Work out the finished part from the listing and answer in its coordinate system (mm). Round coordinates to 2 decimals unless told otherwise and drop trailing zeros. Loops run counter-clockwise (first coordinate to the right, second up) from the corner with the lowest first, then second, coordinate; pieces in that order, holes last. Notation, with made-up numbers: (15.5, 12.25) - (54.5, 12.25) arc R22 ccw to (54.5, 29.25) - close; hole circle Ø4 at (-24, 72.5). An arc over 180 degrees is marked (long way). Answer as CSV lines item,"result". Start each with the question number.
Q1. Section A-A on x = 35.5 is taken. Write down the section's boundary in (y, z), then the cut area to 3 significant figures.
Q2. Section B-B on z = 0.9 is taken. Write down the section's boundary in (x, y), then the cut area to 3 significant figures.
Q3. Section C-C on y = 0 is taken. Write down the section's boundary in (x, z).
Q4. Straight lines are drawn through the part: L1, parallel to Y at x = 21.5, z = 0.85; L2, parallel to X at y = -3.5, z = 1.1; L3, parallel to X at y = 11.5, z = 0.85. For each, find the intervals that lie inside material, in ascending order. Write a range as [from, to].
```python
from build123d import *

# Parameters (mm, degrees)
F0_W     = 87
F0_H     = 59
F1_DEPTH = 2
F2_R     = 17.5
F3_DEPTH = 25
F4_DEPTH = 20
F5_R     = 4


with BuildPart() as f1:
    # F0 (on Top) → F1 (new body)
    with BuildSketch(Plane.XY):
        Rectangle(F0_W, F0_H)
    extrude(amount=F1_DEPTH)

    # F2 (on face) → F3 (cut)
    with BuildSketch(Plane.XY.offset(2)):
        with Locations((21.5, 0)):
            Circle(F2_R)
    extrude(amount=-F3_DEPTH, mode=Mode.SUBTRACT)

    # F4 (add): a face of the model
    f4_faces = [f1.faces().sort_by_distance(p)[0] for p in [
        (-43.5, 0, 1),
    ]]
    extrude(f4_faces, amount=F4_DEPTH)

    # F5
    f5_edges = [f1.edges().sort_by_distance(p)[0] for p in [
        (-63.5, 29.5, 1),
        (-63.5, -29.5, 1),
    ]]
    fillet(f5_edges, radius=F5_R)


solid = f1.part
```
Findings:
1,outline,"(-29.5, 0) - (-10.5, 0) - (-10.5, 2) - (-29.5, 2) - close; (10.5, 0) - (29.5, 0) - (29.5, 2) - (10.5, 2) - close"
1,area,"76.0 mm^2"
2,outline,"(-63.5, -25.5) arc R4 ccw to (-59.5, -29.5) - (43.5, -29.5) - (43.5, 29.5) - (-59.5, 29.5) arc R4 ccw to (-63.5, 25.5) - close; hole circle Ø35 at (21.5, 0)"
2,area,"5,340 mm^2"
3,outline,"(-63.5, 0) - (4, 0) - (4, 2) - (-63.5, 2) - close; (39, 0) - (43.5, 0) - (43.5, 2) - (39, 2) - close"
4,L1,"y = [-29.5, -17.5], [17.5, 29.5]"
4,L2,"x = [-63.5, 4.35], [38.65, 43.5]"
4,L3,"x = [-63.5, 8.31], [34.69, 43.5]"
